The model under review builds one solid part; all positions refer to its coordinate system, in mm. A direction names the side the tool comes from. Coordinates: 2 decimals unless noted, no trailing zeros. Order: outer loops, then holes, each group sorted by start corner. A loop starts at its lowest first (then second) coordinate and runs counter-clockwise, first axis right, second up. Notation, with made-up numbers: M 19.5,-38.5 L 30.5,-38.5 A25 ccw 30.5,-18.5 Z; hole C -10,88.5 d5. An arc over 180 degrees is marked long. Write each question's results on one line, items separated by ' | '.
Autodesk Inventor part; units mm, degrees
ref_plane "Work Plane1" through (-203, 0.4, 290) normal (0, 1, 0) x (1, 0, 0)
ref_plane "Work Plane2" through (-203, 0.6, 290) normal (0, 1, 0) x (1, 0, 0)
ref_plane "YZ Plane" through (0, 0, 0) normal (1, 0, 0) x (0, 1, 0)
ref_plane "Work Plane1" through (-203, 0.4, 290) normal (0, 1, 0) x (1, 0, 0)
sketch "Sketch1" plane through (-203, 0.4, 290) normal (0, 1, 0) x (1, 0, 0)
  arc A0 (133.6, 0) -> (138.4129, 10.1472) centre (133.6, 6.215) ccw
  circle A1 centre (133.6, 6.215) radius 1.675
  circle A2 centre (133.6, 6.215) radius 1.675
  circle A3 centre (133.6, 6.215) radius 1.675
  circle A4 centre (133.6, 6.215) radius 1.675
  arc A5 (133.6, 0) -> (138.4129, 10.1472) centre (133.6, 6.215) ccw
  arc A6 (133.6, 0) -> (138.4129, 10.1472) centre (133.6, 6.215) ccw
  arc A7 (133.6, 0) -> (138.4129, 10.1472) centre (133.6, 6.215) ccw
  circle A8 centre (84.5, 143.475) radius 1.675
  arc A9 (84.5, 138.975) -> (89, 143.475) centre (84.5, 143.475) ccw
  arc A10 (73.455, 136.4093) -> (71.909, 134.5363) centre (73.9075, 134.4612) ccw
  arc A11 (73.455, 136.4093) -> (71.909, 134.5363) centre (73.9075, 134.4612) ccw
  circle A12 centre (5.5, 122.225) radius 1.675
  circle A13 centre (5.5, 122.225) radius 1.675
  circle A14 centre (5.5, 122.225) radius 1.675
  circle A15 centre (5.5, 122.225) radius 1.675
  line L0 (69.5853, 72.7034) -> (71.909, 134.5363)
  line L1 (69.5853, 72.7034) -> (71.909, 134.5363)
  line L2 (69.5853, 72.7034) -> (71.909, 134.5363)
  line L3 (69.5853, 72.7034) -> (71.909, 134.5363)
  circle A16 centre (5.5, 6.215) radius 1.675
  line L4 (0, 0) -> (133.6, 0)
  line L5 (0, 0) -> (133.6, 0)
  line L6 (0, 0) -> (133.6, 0)
  line L7 (0, 0) -> (133.6, 0)
  line L8 (138.4129, 10.1472) -> (70.2502, 71.1379)
  line L9 (138.4129, 10.1472) -> (70.2502, 71.1379)
  line L10 (138.4129, 10.1472) -> (70.2502, 71.1379)
  line L11 (138.4129, 10.1472) -> (70.2502, 71.1379)
  arc A17 (73.455, 136.4093) -> (71.909, 134.5363) centre (73.9075, 134.4612) ccw
  arc A18 (73.455, 136.4093) -> (71.909, 134.5363) centre (73.9075, 134.4612) ccw
  circle A19 centre (5.5, 6.215) radius 1.675
  arc A20 (-2, 2) -> (0, 0) centre (0, 2) ccw
  arc A21 (-2, 2) -> (0, 0) centre (0, 2) ccw
  arc A22 (-2, 2) -> (0, 0) centre (0, 2) ccw
  arc A23 (-2, 2) -> (0, 0) centre (0, 2) ccw
  circle A24 centre (5.5, 6.215) radius 1.675
  circle A25 centre (5.5, 6.215) radius 1.675
  arc A26 (69.5853, 72.7034) -> (70.2502, 71.1379) centre (71.5839, 72.6283) ccw
  arc A27 (69.5853, 72.7034) -> (70.2502, 71.1379) centre (71.5839, 72.6283) ccw
  arc A28 (69.5853, 72.7034) -> (70.2502, 71.1379) centre (71.5839, 72.6283) ccw
  arc A29 (69.5853, 72.7034) -> (70.2502, 71.1379) centre (71.5839, 72.6283) ccw
  arc A30 (84.5, 138.975) -> (89, 143.475) centre (84.5, 143.475) ccw
  circle A31 centre (84.5, 143.475) radius 1.675
  circle A32 centre (84.5, 143.475) radius 1.675
  circle A33 centre (84.5, 143.475) radius 1.675
  arc A34 (84.5, 138.975) -> (89, 143.475) centre (84.5, 143.475) ccw
  arc A35 (84.5, 138.975) -> (89, 143.475) centre (84.5, 143.475) ccw
  line L12 (73.455, 136.4093) -> (84.5, 138.975)
  line L13 (73.455, 136.4093) -> (84.5, 138.975)
  line L14 (73.455, 136.4093) -> (84.5, 138.975)
  line L15 (73.455, 136.4093) -> (84.5, 138.975)
  line L16 (-2, 2) -> (-2, 148.562)
  line L17 (-2, 272.9952) -> (-2, 2)
  line L18 (-2, 148.562) -> (89, 148.562)
  line L19 (89, 143.475) -> (89, 199.525)
  line L20 (89, 148.562) -> (89, 143.475)
  point P0 (203, 290)
  point P1 (-2, 2)
extrude "Extrusion1" add sketch "Sketch1" along normal blind 0.2
ref_plane "Work Plane2" through (-203, 0.6, 290) normal (0, 1, 0) x (1, 0, 0)
sketch "Sketch2" plane through (-203, 0.6, 290) normal (0, 1, 0) x (1, 0, 0)
  line L0 (-2, 272.9952) -> (-2, 2)
  arc A0 (84.5, 138.975) -> (89, 143.475) centre (84.5, 143.475) ccw
  line L1 (-2, 139.0629) -> (89, 143.475)
  circle A1 centre (11.7945, 139.7317) radius 2.5
  circle A2 centre (77.6916, 142.9267) radius 2.5
  circle A3 centre (45.3956, 141.3608) radius 2.5
  point P0 (203, 290)
  dimension "d3" = 5
  dimension "d6" = 5
  dimension "d7" = 5
extrude "Extrusion2" add sketch "Sketch2" along normal blind 1
properties part number "base_main_pcb_p1_itr2"
1) Take a section at C-C on x = -168. State the section outline as (y, z) points, plus the area to 3 significant figures.
Solutions:
outline: M 0.4,141.44 L 0.6,141.44 L 0.6,290 L 0.4,290 Z | area: 29.7 mm2
2) The part is to be moulded in two halves that separate along X. For faces 1 (the cylindrical face through (-127.151, 1.093, 148.763)), 2 (the flat face through (-151, 0.4, 215)), say which applies: pulls with the +X half, pulls with the -X half, needs draft (parallel to the pull), parting line crosses it, or undercut.
Solutions:
face 1: undercut | face 2: needs draft
3) Take a section at A-A on x = -197.5. State the section outline as (y, z) points.
Solutions:
outline: M 0.4,141.44 L 0.6,141.44 L 0.6,166.1 L 0.4,166.1 Z; M 0.4,169.45 L 0.6,169.45 L 0.6,282.11 L 0.4,282.11 Z; M 0.4,285.46 L 0.6,285.46 L 0.6,290 L 0.4,290 Z
4) For pin 1 (4.5 mm diameter, centred on x = -118.5, z = 146.525, fed in from +Y), flat-tipped, find the tip position at first contact; note if it passes through.
Solutions:
pin 1: y = 0.6
5) Take a section at D-D on z = 209. State the section outline as (x, y) points.
Solutions:
outline: M -205,0.4 L -133.1,0.4 L -133.1,0.6 L -205,0.6 Z
6) Take a section at B-B on y = 1.3. State the section outline as (x, z) points, plus the area to 3 significant figures.
Solutions:
outline: C -191.21,150.27 d5; C -157.6,148.64 d5; C -125.31,147.07 d5 | area: 58.9 mm2
7) For faces 3 (the flat face through (-158, 1.6, 149)), 4 (the cylindrical face through (-156.26, 1.093, 150.747)), list the 3-axis set-ups (+Z, -Z, +X, -X, +Y, -Y) from which the entire face can be reached by the end or side of a thin tool; tool diameter is ignored.
Solutions:
face 3: +Z, -Z, +X, -X, +Y | face 4: +Y
8) To check wall thickness, follow line 1 along Z through (x, y) = (-197.5, 0.5); line 2 along Z through (x, y) = (-118.5, 0.5) (3 decimals); line 3 along Y through (x, z) = (-109.5, 269). State the ranges of each line that lie inside material, in increasing order.
Solutions:
line 1: 141.44 to 166.1, 169.45 to 282.11, 285.46 to 290 | line 2: 141.438 to 144.85, 148.2 to 151.025, 231.613 to 290 | line 3: 0.4 to 0.6
